CAD build for the part. Positions are in the model's coordinates, mm. A direction names the side the tool comes from. Coordinates: 2 decimals unless noted, no trailing zeros. Write each loop counter-clockwise with the first axis right and the second up, starting at its lowest first coordinate (ties: lowest second). Pieces come first, ordered by that corner, then holes.
```python
from build123d import *

# Parameters (mm, degrees)
PAD_DEPTH       = 40
SKETCH001_R     = 1.65
POCKET_DEPTH    = 13.501
SKETCH002_R     = 10.6
POCKET001_DEPTH = 30.4
SKETCH003_R     = 10.6
POCKET002_DEPTH = 30.4
FILLET_R        = 5
CHAMFER_SIZE    = 1
SKETCH004_R     = 3.1
POCKET003_DEPTH = 5


with BuildPart() as part:
    # Sketch → Pad (new body, symmetric)
    with BuildSketch(Plane.XY):
        with BuildLine():
            Line((-20.5, -13.5), (20.5, -13.5))
            Line((20.5, -13.5), (20.5, 0))
            Line((20.5, 0), (6.5, 0))
            ThreePointArc((-6.5, 0), (0, -6.5), (6.5, 0))
            Line((-6.5, 0), (-20.5, 0))
            Line((-20.5, 0), (-20.5, -13.5))
        make_face()
    extrude(amount=PAD_DEPTH, both=True)

    # Sketch001 → Pocket (cut, through all)
    with BuildSketch(Plane.XZ):
        with Locations((-15.5, 35)):
            Circle(SKETCH001_R)
        with Locations((-15.5, 0)):
            Circle(SKETCH001_R)
        with Locations((-15.5, -35)):
            Circle(SKETCH001_R)
        with Locations((15.5, -35)):
            Circle(SKETCH001_R)
        with Locations((15.5, 0)):
            Circle(SKETCH001_R)
        with Locations((15.5, 35)):
            Circle(SKETCH001_R)
    extrude(amount=POCKET_DEPTH, mode=Mode.SUBTRACT)

    # Sketch002 (on DatumPlane) → Pocket001 (cut)
    with BuildSketch(Plane.XY.offset(35)):
        Circle(SKETCH002_R)
    extrude(amount=-POCKET001_DEPTH, mode=Mode.SUBTRACT)

    # Sketch003 (on DatumPlane) → Pocket002 (cut)
    with BuildSketch(Plane.XY.offset(-35)):
        Circle(SKETCH003_R)
    extrude(amount=POCKET002_DEPTH, mode=Mode.SUBTRACT)

    # Fillet
    fillet_edges = [part.edges().sort_by_distance(p)[0] for p in [
        (-20.5, -6.75, 40),
        (20.5, -6.75, 40),
    ]]
    fillet(fillet_edges, radius=FILLET_R)

    # Chamfer
    chamfer_edges = [part.edges().sort_by_distance(p)[0] for p in [
        (-20.5, -13.5, -2.5),
        (0, -13.5, -40),
    ]]
    chamfer(chamfer_edges, length=CHAMFER_SIZE)

    # Sketch004 (on Face1 of Chamfer) → Pocket003 (cut)
    with BuildSketch(Plane.XZ.offset(13.5)):
        with Locations((-15.5, 35)):
            Circle(SKETCH004_R)
        with Locations((-15.5, 0)):
            Circle(SKETCH004_R)
        with Locations((-15.5, -35)):
            Circle(SKETCH004_R)
        with Locations((15.5, 35)):
            Circle(SKETCH004_R)
        with Locations((15.5, 0)):
            Circle(SKETCH004_R)
        with Locations((15.5, -35)):
            Circle(SKETCH004_R)
    extrude(amount=-POCKET003_DEPTH, mode=Mode.SUBTRACT)


solid = part.part
```
Item 1: Saw through at C-C, the plane x = 0. Write the cut outline in (y, z).
Item 2: Flat gauge pins, fed straight in: pin 1 Ø3 at (x, z) = (14.5, 0) entering from -Y; pin 2 Ø2.5 at (x, z) = (15.5, 35) entering from +Y; pin 3 Ø12 at (x, z) = (1.5, 28.5) entering from +Y. Where does each tip first touch, or does it go through?
Item 3: Which spindle directions (+Z, -Z, +X, -X, +Y, -Y) get a long thin tool onto all of the face, cutting with end or side? Do faces 1 (the cylindrical face through (-0.1, -6.5, 37.5)), 2 (the flat face through (0, -8, 35)), 3 (the flat face through (-14, -8.5, 34)). Say none if no direction does.
Item 4: Saw through at A-A, the plane y = -5.25. State how many separate pieces and enclosed holes the cut face has, and give its area (3 significant figures).
Item 5: Two-plate mould, pull along Z, no slides. Class faces 4 (the conical face through (18.563, -13.215, 37.996)), 5 (the flat face through (-13, 0, 1)), 6 (the flat face through (17, -8.5, 34)): +Z half, -Z half, draft (parallel to the pull), parting line (faces both ways), or undercut.
Item 6: Wall check: line 1 along Z through (x, y) = (-15.5, -10.9); line 2 along Z through (x, y) = (5, -5.5); line 3 along Z through (x, y) = (15.5, -5). Give the ranges that are in metal, low to high.
Item 7: Saw through at B-B, the plane z = -25.5. Write the cut outline in (x, y).
Working result:
1. outline: (-13.5, -39) - (-12.5, -40) - (-6.5, -40) - (-6.5, -35) - (-10.6, -35) - (-10.6, -4.6) - (-6.5, -4.6) - (-6.5, 4.6) - (-10.6, 4.6) - (-10.6, 35) - (-6.5, 35) - (-6.5, 40) - (-12.5, 40) - (-13.5, 39) - close
2. pin 1: stops at y = -8.5
2. pin 2: passes through
2. pin 3: stops at y = -7.49
3. face 1: +Z, -Z, +Y
3. face 2: +Y
3. face 3: -Y
4. separate pieces: 2
4. enclosed holes: 6
4. area: 1,950 mm2
5. face 4: +Z half
5. face 5: draft
5. face 6: undercut
6. line 1: z = -40 to -38.1, -31.9 to -3.1, 3.1 to 31.9, 38.1 to 40
6. line 2: z = -40 to -35, -4.6 to 4.6, 35 to 40
6. line 3: z = -40 to -36.65, -33.35 to -1.65, 1.65 to 33.35, 36.65 to 40
7. outline: (-20.5, -12.5) - (-19.5, -13.5) - (19.5, -13.5) - (20.5, -12.5) - (20.5, 0) - (10.6, 0) arc R10.6 cw to (-10.6, 0) - (-20.5, 0) - close
